Check sheet for the modelled part. Datum: model origin and axes. Units: mm. A direction names the side the tool comes from. Coordinates: 2 decimals unless noted, no trailing zeros. Order: outer loops, then holes, each group sorted by start corner. A loop starts at its lowest first (then second) coordinate and runs counter-clockwise, first axis right, second up.
from build123d import *

# Parameters (mm, degrees)
EXTRUDE_1_DEPTH     = 60
CUT_EXTRUDE_1_REACH = 95
SKETCH_2_R          = 4
FILLET_1_R          = 10
CUT_EXTRUDE_2_REACH = 95
SKETCH_3_R          = 4


with BuildPart() as part:
    # 草图1 → 凸台-拉伸1 (new body)
    with BuildSketch(Plane.XY):
        with BuildLine():
            Line((-42.5, 0), (-42.5, 61))
            ThreePointArc((-42.5, 61), (-41.328427125, 63.828427125), (-38.5, 65))
            Line((-38.5, 65), (38.5, 65))
            ThreePointArc((38.5, 65), (41.328427125, 63.828427125), (42.5, 61))
            Line((42.5, 61), (42.5, 30))
            Line((42.5, 30), (46.5, 30))
            Line((46.5, 30), (46.5, 61))
            ThreePointArc((46.5, 61), (44.156854249, 66.656854249), (38.5, 69))
            Line((38.5, 69), (-38.5, 69))
            ThreePointArc((-38.5, 69), (-44.156854249, 66.656854249), (-46.5, 61))
            Line((-46.5, 61), (-46.5, 0))
            Line((-46.5, 0), (-42.5, 0))
        make_face()
    extrude(amount=EXTRUDE_1_DEPTH)

    # 草图2 → 切除-拉伸1 (cut, up to next)
    with BuildSketch(Plane.ZY.offset(46.5), mode=Mode.PRIVATE) as cut_extrude_1_sk1:
        with Locations((15, 30)):
            Circle(SKETCH_2_R)
    cut_extrude_1_tool1 = extrude(cut_extrude_1_sk1.sketch, amount=-CUT_EXTRUDE_1_REACH, mode=Mode.PRIVATE) & part.part
    add(cut_extrude_1_tool1.solids().sort_by_distance((-46.5, 30, 15))[0], mode=Mode.SUBTRACT)
    # 草图2 → 切除-拉伸1 (cut, up to next)
    with BuildSketch(Plane.ZY.offset(46.5), mode=Mode.PRIVATE) as cut_extrude_1_sk2:
        with Locations((45, 30)):
            Circle(SKETCH_2_R)
    cut_extrude_1_tool2 = extrude(cut_extrude_1_sk2.sketch, amount=-CUT_EXTRUDE_1_REACH, mode=Mode.PRIVATE) & part.part
    add(cut_extrude_1_tool2.solids().sort_by_distance((-46.5, 30, 45))[0], mode=Mode.SUBTRACT)

    # 圆角1
    fillet_1_edges = [part.edges().sort_by_distance(p)[0] for p in [
        (44.5, 30, 0),
        (-44.5, 0, 0),
        (44.5, 30, 60),
        (-44.5, 0, 60),
    ]]
    fillet(fillet_1_edges, radius=FILLET_1_R)

    # 草图3 → 切除-拉伸2 (cut, up to next)
    with BuildSketch(Plane(origin=(46.5, 0, 0), x_dir=(0, 0, -1), z_dir=(1, 0, 0)), mode=Mode.PRIVATE) as cut_extrude_2_sk1:
        with Locations((-45, 45)):
            Circle(SKETCH_3_R)
    cut_extrude_2_tool1 = extrude(cut_extrude_2_sk1.sketch, amount=-CUT_EXTRUDE_2_REACH, mode=Mode.PRIVATE) & part.part
    add(cut_extrude_2_tool1.solids().sort_by_distance((46.5, 45, 45))[0], mode=Mode.SUBTRACT)
    # 草图3 → 切除-拉伸2 (cut, up to next)
    with BuildSketch(Plane(origin=(46.5, 0, 0), x_dir=(0, 0, -1), z_dir=(1, 0, 0)), mode=Mode.PRIVATE) as cut_extrude_2_sk2:
        with Locations((-15, 45)):
            Circle(SKETCH_3_R)
    cut_extrude_2_tool2 = extrude(cut_extrude_2_sk2.sketch, amount=-CUT_EXTRUDE_2_REACH, mode=Mode.PRIVATE) & part.part
    add(cut_extrude_2_tool2.solids().sort_by_distance((46.5, 45, 15))[0], mode=Mode.SUBTRACT)


solid = part.part
(1) Go/stop test with flat-tipped pins: P1, Ø18, axis at y = 27, z = 40, coming from the +X side; P2, Ø5, axis at y = 45, z = 15, coming from the +X side; P3, Ø1.2, axis at x = 44.5, z = 28.5, coming from the -Y side; P4, Ø12, axis at x = -17.5, z = 16.5, coming from the -Y side. Record where each tip stops, or that it passes through.
Filled in:
P1: stops at x = 46.5
P2: stops at x = -42.5
P3: stops at y = 30
P4: stops at y = 65
(2) Cross-section at C-C (y = 54.5). Enter the section's corners in (x, z), and give its area (3 significant figures).
Filled in:
outline: (-46.5, 0) - (-42.5, 0) - (-42.5, 60) - (-46.5, 60) - close; (42.5, 0) - (46.5, 0) - (46.5, 60) - (42.5, 60) - close
area: 480 mm2
(3) Cross-section at A-A (z = 45). Enter the section's corners in (x, y), and give its area (3 significant figures).
Filled in:
outline: (-46.5, 0) - (-42.5, 0) - (-42.5, 26) - (-46.5, 26) - close; (-46.5, 34) - (-42.5, 34) - (-42.5, 61) arc R4 cw to (-38.5, 65) - (38.5, 65) arc R4 cw to (42.5, 61) - (42.5, 49) - (46.5, 49) - (46.5, 61) arc R8 ccw to (38.5, 69) - (-38.5, 69) arc R8 ccw to (-46.5, 61) - close; (42.5, 30) - (46.5, 30) - (46.5, 41) - (42.5, 41) - close
area: 687 mm2
(4) Tool access check on faces 1 (the cylindrical face through (44.5, 42.6, 18.2)), 2 (the cylindrical face through (-44.528, 33.966, 14.479)), 3 (the cylindrical face through (44.53, 33.01, 57.15)), 4 (the flat face through (44, 30, 30)). Record the directions out of +Z, -Z, +X, -X, +Y, -Y that give a thin tool (end or side, any length) a straight path to the whole face; none if there is none.
Filled in:
face 1: +X
face 2: -X
face 3: +Z, +X, -Y
face 4: +Z, -Z, +X, -Y
(5) Cross-section at B-B (y = 45). Enter the section's corners in (x, z).
Filled in:
outline: (-46.5, 0) - (-42.5, 0) - (-42.5, 60) - (-46.5, 60) - close; (42.5, 0) - (46.5, 0) - (46.5, 11) - (42.5, 11) - close; (42.5, 19) - (46.5, 19) - (46.5, 41) - (42.5, 41) - close; (42.5, 49) - (46.5, 49) - (46.5, 60) - (42.5, 60) - close
(6) Thickness scan on probe 1 along X at (y, z) = (58, 36.5); probe 2 along X at (y, z) = (12, 36); probe 3 along Y at (x, z) = (-33, 52.5). Record the ranges inside material, lowest first.
Filled in:
probe 1: x = -46.5 to -42.5, 42.5 to 46.5
probe 2: x = -46.5 to -42.5
probe 3: y = 65 to 69
(7) Cross-section at D-D (z = 27). Enter the section's corners in (x, y), and give its area (3 significant figures).
Filled in:
outline: (-46.5, 0) - (-42.5, 0) - (-42.5, 61) arc R4 cw to (-38.5, 65) - (38.5, 65) arc R4 cw to (42.5, 61) - (42.5, 30) - (46.5, 30) - (46.5, 61) arc R8 ccw to (38.5, 69) - (-38.5, 69) arc R8 ccw to (-46.5, 61) - close
area: 751 mm2
(8) Release check for a two-part mould opening along X. For faces 5 (the cylindrical face through (-44.094, 66.719, 29.58)), 6 (the flat face through (-1, 65, 30)), 7 (the cylindrical face through (44.5, 42.6, 48.2)), 8 (the flat face through (46.5, 45, 30)) record: +X half, -X half, draft (parallel to the pull), parting line (faces both ways), or undercut.
Filled in:
face 5: -X half
face 6: undercut
face 7: draft
face 8: +X half
